Build history of the part. All positions in model axes, mm. Coordinates: 2 decimals unless noted, no trailing zeros. Loops run counter-clockwise (first coordinate to the right, second up) from the corner with the lowest first, then second, coordinate; pieces in that order, holes last.
Item 1: Flat gauge pin, fed straight in: pin 1 (1 mm diameter, centred on x = 43.5, y = 16.5, fed in from -Z). Where does the tip first touch, or does it go through?
Item 2: Cut at C-C (x = -12). List the corners of the cut face in (y, z), and give its area (3 significant figures).
Item 3: Drill centre lines: line 1 along X through (y, z) = (-6.5, 1.5); line 2 along Y through (x, z) = (-2, 1.95); line 3 along Y through (x, z) = (42, 0.3). Where is each one in solid material? Low to high.
Item 4: Cut at B-B (z = 1). List the corners of the cut face in (x, y), and give its area (3 significant figures).
Item 5: Cut at A-A (y = 2). List the corners of the cut face in (x, z).
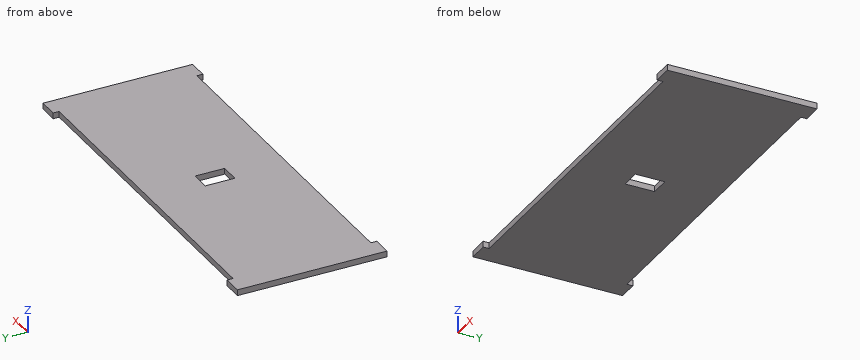
from build123d import *

# Parameters (mm, degrees)
ESBO_O1_W                = 10
ESBO_O1_H                = 3
ESBO_O1_W_2              = 190
ESBO_O1_H_2              = 70
RESSALTO_EXTRUS_O1_DEPTH = 3
ESBO_O2_W                = 10
ESBO_O2_H                = 15
CORTE_EXTRUS_O1_DEPTH    = 10


with BuildPart() as part:
    # Esboço1 → Ressalto-extrusão1 (new body)
    with BuildSketch(Plane.XY):
        with Locations((-90, -36.5)):
            Rectangle(ESBO_O1_W, ESBO_O1_H)
        with Locations((-90, 36.5)):
            Rectangle(ESBO_O1_W, ESBO_O1_H)
        Rectangle(ESBO_O1_W_2, ESBO_O1_H_2)
        with Locations((90, 36.5)):
            Rectangle(ESBO_O1_W, ESBO_O1_H)
        with Locations((90, -36.5)):
            Rectangle(ESBO_O1_W, ESBO_O1_H)
    extrude(amount=RESSALTO_EXTRUS_O1_DEPTH)

    # Esboço2 → Corte-extrusão1 (cut)
    with BuildSketch(Plane.XY.offset(3)):
        Rectangle(ESBO_O2_W, ESBO_O2_H)
    extrude(amount=-CORTE_EXTRUS_O1_DEPTH, mode=Mode.SUBTRACT)


solid = part.part
Filled sheet:
1. pin 1: stops at z = 0
2. outline: (-35, 0) - (35, 0) - (35, 3) - (-35, 3) - close
2. area: 210 mm2
3. line 1: x = -95 to -5, 5 to 95
3. line 2: y = -35 to -7.5, 7.5 to 35
3. line 3: y = -35 to 35
4. outline: (-95, -38) - (-85, -38) - (-85, -35) - (85, -35) - (85, -38) - (95, -38) - (95, 38) - (85, 38) - (85, 35) - (-85, 35) - (-85, 38) - (-95, 38) - close; hole (-5, -7.5) - (5, -7.5) - (5, 7.5) - (-5, 7.5) - close
4. area: 13,300 mm2
5. outline: (-95, 0) - (-5, 0) - (-5, 3) - (-95, 3) - close; (5, 0) - (95, 0) - (95, 3) - (5, 3) - close
